```python
from build123d import *

# Parameters (mm, degrees)
SKETCH_1_W          = 25
SKETCH_1_H          = 23
EXTRUDE_1_DEPTH     = 12
CUT_EXTRUDE_START   = 1
SKETCH_2_W          = 25
SKETCH_2_H          = 21
CUT_EXTRUDE_1_DEPTH = 11
EXTRUDE_START       = 12
SKETCH_6_W          = 25
SKETCH_6_H          = 23
EXTRUDE_3_DEPTH     = 1
CUT_EXTRUDE_START_2 = 13
SKETCH_8_R          = 9.75
CUT_EXTRUDE_2_DEPTH = 1
SKETCH_10_W         = 25
SKETCH_10_H         = 23
CUT_EXTRUDE_4_DEPTH = 12


with BuildPart() as part:
    # 스케치1 → 보스-돌출1 (new body)
    with BuildSketch(Plane(origin=(0, 0, 0), x_dir=(1, 0, 0), z_dir=(0, 1, 0))):
        Rectangle(SKETCH_1_W, SKETCH_1_H)
    extrude(amount=EXTRUDE_1_DEPTH)

    # 스케치2 → 컷-돌출1 (cut)
    with BuildSketch(Plane(origin=(0, 0, 0), x_dir=(1, 0, 0), z_dir=(0, 1, 0)).offset(CUT_EXTRUDE_START)):
        with Locations((1, 0)):
            Rectangle(SKETCH_2_W, SKETCH_2_H)
    extrude(amount=CUT_EXTRUDE_1_DEPTH, mode=Mode.SUBTRACT)

    # 스케치10 → 컷-돌출4 (cut)
    with BuildSketch(Plane.XZ):
        Rectangle(SKETCH_10_W, SKETCH_10_H)
    extrude(amount=-CUT_EXTRUDE_4_DEPTH, mode=Mode.SUBTRACT)


with BuildPart() as body_2:
    # 스케치6 → 보스-돌출3 (new body)
    with BuildSketch(Plane(origin=(0, 0, 0), x_dir=(1, 0, 0), z_dir=(0, 1, 0)).offset(EXTRUDE_START)):
        Rectangle(SKETCH_6_W, SKETCH_6_H)
    extrude(amount=EXTRUDE_3_DEPTH)

    # 스케치8 → 컷-돌출2 (cut)
    with BuildSketch(Plane(origin=(0, 0, 0), x_dir=(1, 0, 0), z_dir=(0, 1, 0)).offset(CUT_EXTRUDE_START_2)):
        with Locations(Location((0.25, 0, 0), (0, 0, 270))):
            Circle(SKETCH_8_R)
    extrude(amount=-CUT_EXTRUDE_2_DEPTH, mode=Mode.SUBTRACT)


solid = body_2.part
```
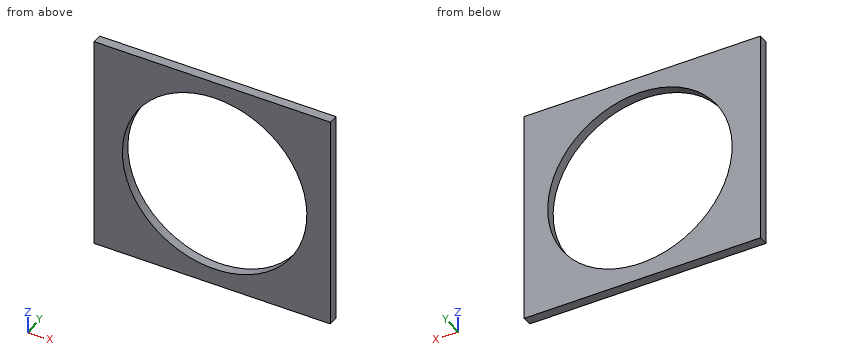
The model under review builds one solid part; all positions refer to its coordinate system, in mm. Round coordinates to 2 decimals unless told otherwise and drop trailing zeros. Write each loop counter-clockwise with the first axis right and the second up, starting at its lowest first coordinate (ties: lowest second). Pieces come first, ordered by that corner, then holes. Notation, with made-up numbers: (36, 71.5) - (91, 71.5) arc R26 ccw to (91, 99.5) - close; hole circle Ø3 at (56.5, 1). An arc over 180 degrees is marked (long way). Use one line per item in the form item = value.
Q1. For line 1 (X direction, y = 12.85, z = 0); line 2 (Z direction, x = 0.5, y = 12.65); line 3 (X direction, y = 12.9, z = 4), list the stretches that pass through material, from the lowest coordinate up. Write a range as [from, to].
Answer key:
line_1 = [-12.5, -9.5], [10, 12.5]
line_2 = [-11.5, -9.75], [9.75, 11.5]
line_3 = [-12.5, -8.64], [9.14, 12.5]
Q2. Consider section B-B (y = 12.5). State the section outline as (x, z) points.
Answer key:
outline = (-12.5, -11.5) - (12.5, -11.5) - (12.5, 11.5) - (-12.5, 11.5) - close; hole circle Ø19.5 at (0.25, 0)
Q3. Consider section C-C (z = 0). State the section outline as (x, y) points.
Answer key:
outline = (-12.5, 12) - (-9.5, 12) - (-9.5, 13) - (-12.5, 13) - close; (10, 12) - (12.5, 12) - (12.5, 13) - (10, 13) - close
Q4. Consider section A-A (x = 0.25). State the section outline as (y, z) points.
Answer key:
outline = (12, -11.5) - (13, -11.5) - (13, -9.75) - (12, -9.75) - close; (12, 9.75) - (13, 9.75) - (13, 11.5) - (12, 11.5) - close
